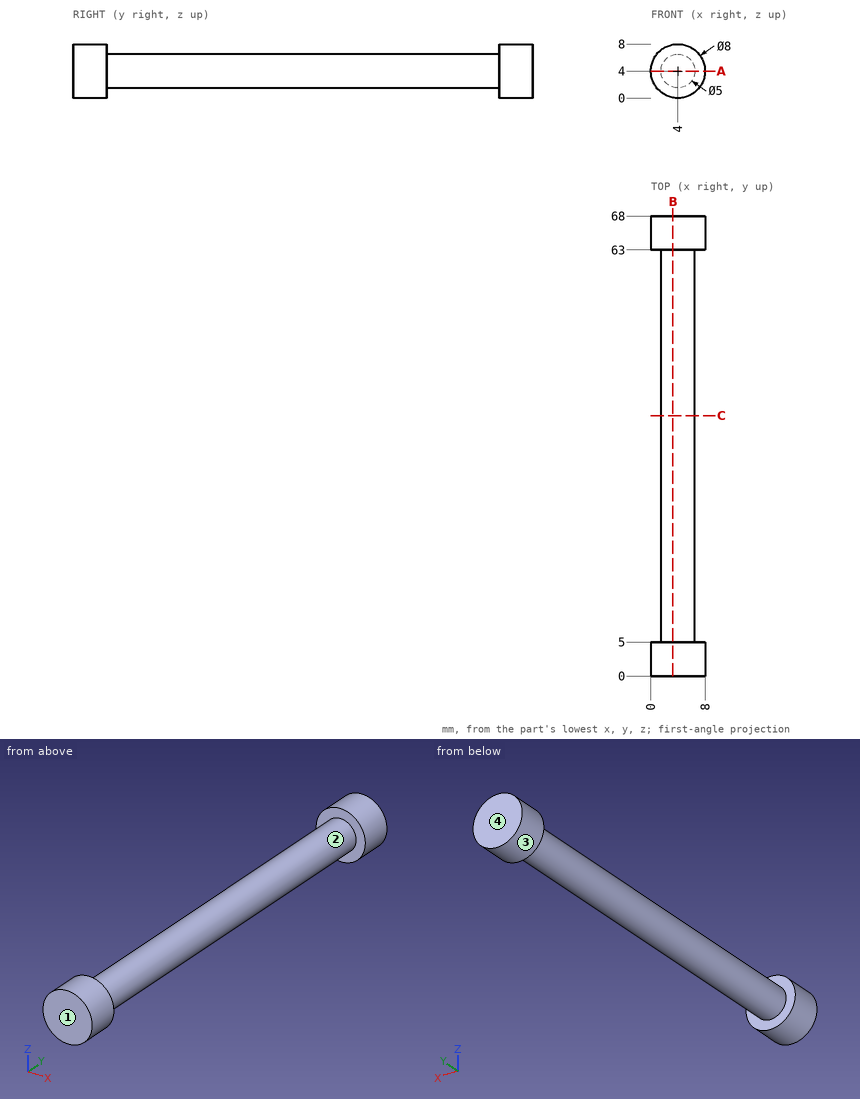
Verification items for this drawing (mm, ordinates from the low corner). Round coordinates to 2 decimals unless told otherwise and drop trailing zeros. Loops run counter-clockwise (first coordinate to the right, second up) from the corner with the lowest first, then second, coordinate; pieces in that order, holes last. Notation, with made-up numbers: (-11.75, -35.75) - (8.25, -35.75) arc R14 cw to (8.25, -19.75) - close; hole circle Ø6 at (-35, 88.5). An arc over 180 degrees is marked (long way). Answer as CSV lines item,"result". Start each with the question number.
Item 1: Section check A-A (z = 4). Record the boundary of the cut face in (x, y), and give its area (3 significant figures).
Item 2: Scan lines: line 1 (Y direction, x = 1.75, z = 2.25); line 2 (X direction, y = 20, z = 4); line 3 (X direction, y = 12, z = 2.75). Record each from-to range of solid material in increasing order. Write a range as [from, to].
Item 3: Release check for a two-part mould opening along Y. For the marked faces 1, 2, 3 and 4 record: +Y half, -Y half, draft (parallel to the pull), parting line (faces both ways), or undercut.
Item 4: Section check B-B (x = 3.25). Record the boundary of the cut face in (y, z), and give its area (3 significant figures).
Item 5: Depth check by flat-ended pin: P1, Ø1.5, axis at y = 10.5, z = 6.5, coming from the +X side; P2, Ø1, axis at x = 6.5, z = 2, coming from the -Y side; P3, Ø4, axis at y = 52.5, z = 5.5, coming from the -X side; P4, Ø3, axis at y = 32, z = 4.5, coming from the +X side. Enter the tip coordinate at first touch or a pass-through.
Item 6: Section check C-C (y = 38.5). Record the boundary of the cut face in (x, z), and give its area (3 significant figures).
Report:
1,outline,"(0, 0) - (8, 0) - (8, 5) - (6.5, 5) - (6.5, 63) - (8, 63) - (8, 68) - (0, 68) - (0, 63) - (1.5, 63) - (1.5, 5) - (0, 5) - close"
1,area,"370 mm2"
2,line 1,"y = [0, 5], [63, 68]"
2,line 2,"x = [1.5, 6.5]"
2,line 3,"x = [1.83, 6.17]"
3,face 1,"-Y half"
3,face 2,"undercut"
3,face 3,"draft"
3,face 4,"+Y half"
4,outline,"(0, 0.07) - (5, 0.07) - (5, 1.62) - (63, 1.62) - (63, 0.07) - (68, 0.07) - (68, 7.93) - (63, 7.93) - (63, 6.38) - (5, 6.38) - (5, 7.93) - (0, 7.93) - close"
4,area,"355 mm2"
5,P1,"stops at x = 5.79"
5,P2,"stops at y = 0"
5,P3,"stops at x = 1.5"
5,P4,"stops at x = 6.5"
6,outline,"circle Ø5 at (4, 4)"
6,area,"19.6 mm2"
